The model under review builds one solid part; all positions refer to its coordinate system, in mm. A direction names the side the tool comes from. Round coordinates to 2 decimals unless told otherwise and drop trailing zeros. Loops run counter-clockwise (first coordinate to the right, second up) from the corner with the lowest first, then second, coordinate; pieces in that order, holes last. Notation, with made-up numbers: M 24,10.5 L 71,10.5 A12 ccw 71,15.5 Z; hole C 63,-23 d1. An arc over 180 degrees is marked long. Return JSON: item names as keys, results as strings. Group by question number.
Q1. Consider section B-B (z = 32.75). State the section outline as (x, y) points.
Q2. For faces 5 (the face through (8.804, 24.921, 27.985)), 6 (the face through (25, 16.722, 37)), 7 (the face through (20.218, 24.937, 35.375)), 8 (the face through (13, 24.222, 30)), list the 3-axis set-ups (+Z, -Z, +X, -X, +Y, -Y) from which the entire face can be reached by the end or side of a thin tool; tool diameter is ignored.
Q3. Consider section A-A (y = 18.25). State the section outline as (x, z) points, and give its area (3 significant figures).
Q4. Clearance check with flat-ended pins moving along their axes: pin 1 Ø0.7 at (x, y) = (4.5, 16) entering from -Z; pin 2 Ø4.5 at (x, z) = (15, 34.5) entering from -Y; pin 3 Ø3 at (y, z) = (19, 34.5) entering from +X; pin 4 Ø1.6 at (x, z) = (5.06, 37.89) entering from -Y. State where each tip first meets the part, or that it passes through.
Q5. To check wall thickness, follow line 1 along X through (y, z) = (22, 32); line 2 along Y through (x, z) = (16, 30.75); line 3 along Y through (x, z) = (15, 32.25). State the ranges of each line that lie inside material, in increasing order.
Q6. Consider section C-C (y = 16). State the section outline as (x, z) points, and give its area (3 significant figures).
Q7. Draft analysis for pull direction X (two halves, no side actions). For faces 1 (the face through (8.804, 24.921, 35.375)), 2 (the face through (20.519, 20, 34)), 3 (the face through (7.519, 20, 34)), 4 (the face through (14, 26, 40.09)), state which applies: pulls with the +X half, pulls with the -X half, needs draft (parallel to the pull), parting line crosses it, or undercut.
Q8. Consider section D-D (z = 38.5). State the section outline as (x, y) points, and give its area (3 significant figures).
from build123d import *

# Parameters (mm, degrees)
BOSS_EXTRUDE1_DEPTH = 12.5
SKETCH3_R           = 1
CUT_EXTRUDE1_DEPTH  = 49.99745314
FILLET1_R           = 1
SKETCH4_W           = 12
SKETCH4_H           = 2.4
BOSS_EXTRUDE2_DEPTH = 1
CAVITY2_START       = 28.390407362
CAVITY2_DEPTH       = 2.4
FILLET2_R           = 1
SKETCH5_W           = 5
SKETCH5_H           = 8
CUT_EXTRUDE2_DEPTH  = 49.99745314
FILLET3_R           = 1


# Read off the part's stored shape, not the designer's step: Cavity2
with BuildPart() as part:
    # Sketch2 → Boss-Extrude1 (new body)
    with BuildSketch(Plane.XY.offset(40.090407362)):
        Polygon((8.51904319, 15.222118346), (8.51904319, 25.222118346), (20.51904319, 25.222118346), (20.51904319, 15.222118346), (21.51904319, 15.222118346), (26.51904319, 15.222118346), (26.51904319, 16.722118346), (21.51904319, 16.722118346), (21.51904319, 26.222118346), (7.51904319, 26.222118346), (7.51904319, 16.722118346), (2.51904319, 16.722118346), (2.51904319, 15.222118346), (7.51904319, 15.222118346), align=None)
    extrude(amount=-BOSS_EXTRUDE1_DEPTH)

    # Sketch3 → Cut-Extrude1 (cut, through all)
    with BuildSketch(Plane(origin=(0, 16.722118346, 0), x_dir=(1, 0, 0), z_dir=(0, 1, 0))):
        with Locations(Location((5.05904319, -37.891330821, 0), (0, 0, 270))):
            Circle(SKETCH3_R)
        with Locations(Location((23.97904319, -37.891330821, 0), (0, 0, 270))):
            Circle(SKETCH3_R)
    extrude(amount=-CUT_EXTRUDE1_DEPTH, mode=Mode.SUBTRACT)

    # Fillet1
    fillet1_edges = [part.edges().sort_by_distance(p)[0] for p in [
        (8.51904319, 25.222118346, 33.840407362),
        (20.51904319, 25.222118346, 33.840407362),
    ]]
    fillet(fillet1_edges, radius=FILLET1_R)

    # Sketch4 → Boss-Extrude2 (add)
    with BuildSketch(Plane.XZ.offset(-25.222118346)):
        with Locations((14.51904319, 29.590407362)):
            Rectangle(SKETCH4_W, SKETCH4_H)
    extrude(amount=BOSS_EXTRUDE2_DEPTH)

    # Cavity2 outline → Cavity2 (cut)
    with BuildSketch(Plane.XY.offset(CAVITY2_START)):
        with BuildLine():
            Line((17.186568025, 24.222118346), (19.451518355, 24.222118346))
            ThreePointArc((19.451518355, 24.222118346), (18.31904319, 24.672118346), (17.186568025, 24.222118346))
        make_face()
    extrude(amount=CAVITY2_DEPTH, mode=Mode.SUBTRACT)

    # Fillet2
    fillet2_edges = [part.edges().sort_by_distance(p)[0] for p in [
        (21.51904319, 26.222118346, 33.840407362),
        (7.51904319, 26.222118346, 33.840407362),
    ]]
    fillet(fillet2_edges, radius=FILLET2_R)

    # Sketch5 → Cut-Extrude2 (cut, through all)
    with BuildSketch(Plane(origin=(0, 16.722118346, 0), x_dir=(1, 0, 0), z_dir=(0, 1, 0))):
        with Locations((5.01904319, -31.590407362)):
            Rectangle(SKETCH5_W, SKETCH5_H)
        with Locations((24.01904319, -31.590407362)):
            Rectangle(SKETCH5_W, SKETCH5_H)
    extrude(amount=-CUT_EXTRUDE2_DEPTH, mode=Mode.SUBTRACT)

    # Fillet3
    fillet3_edges = [part.edges().sort_by_distance(p)[0] for p in [
        (21.51904319, 16.722118346, 37.840407362),
        (7.51904319, 16.722118346, 37.840407362),
    ]]
    fillet(fillet3_edges, radius=FILLET3_R)


solid = part.part
Values:
{
 "1": {"outline": "M 7.52,15.22 L 8.52,15.22 L 8.52,24.22 A1 cw 9.52,25.22 L 19.52,25.22 A1 cw 20.52,24.22 L 20.52,15.22 L 21.52,15.22 L 21.52,25.22 A1 ccw 20.52,26.22 L 8.52,26.22 A1 ccw 7.52,25.22 Z"},
 "2": {"face 5": "-Z, -Y", "face 6": "+Z, -Z, +X, +Y", "face 7": "+Z, -Y", "face 8": "+Z, -Z, -Y"},
 "3": {"outline": "M 7.52,27.59 L 8.52,27.59 L 8.52,40.09 L 7.52,40.09 Z; M 20.52,27.59 L 21.52,27.59 L 21.52,40.09 L 20.52,40.09 Z", "area": "25.0 mm2"},
 "4": {"pin 1": "stops at z = 35.59", "pin 2": "stops at y = 25.22", "pin 3": "stops at x = 21.52", "pin 4": "passes through"},
 "5": {"line 1": "x = 7.52 to 8.52, 20.52 to 21.52", "line 2": "y = 24.22 to 26.22", "line 3": "y = 25.22 to 26.22"},
 "6": {"outline": "M 2.52,35.59 L 7.52,35.59 L 7.52,27.59 L 8.52,27.59 L 8.52,40.09 L 2.52,40.09 Z; M 20.52,27.59 L 21.52,27.59 L 21.52,35.59 L 26.52,35.59 L 26.52,40.09 L 20.52,40.09 Z; hole C 5.06,37.89 d2; hole C 23.98,37.89 d2", "area": "63.7 mm2"},
 "7": {"face 1": "undercut", "face 2": "undercut", "face 3": "pulls with the -X half", "face 4": "needs draft"},
 "8": {"outline": "M 2.52,15.22 L 4.27,15.22 L 4.27,16.72 L 2.52,16.72 Z; M 5.85,15.22 L 8.52,15.22 L 8.52,24.22 A1 cw 9.52,25.22 L 19.52,25.22 A1 cw 20.52,24.22 L 20.52,15.22 L 23.19,15.22 L 23.19,16.72 L 22.52,16.72 A1 cw 21.52,17.72 L 21.52,25.22 A1 ccw 20.52,26.22 L 8.52,26.22 A1 ccw 7.52,25.22 L 7.52,17.72 A1 cw 6.52,16.72 L 5.85,16.72 Z; M 24.77,15.22 L 26.52,15.22 L 26.52,16.72 L 24.77,16.72 Z", "area": "44.7 mm2"}
}
